Could you check a few things on this model? Use its own coordinates, in mm. Round coordinates to 2 decimals unless told otherwise and drop trailing zeros. Write each loop counter-clockwise with the first axis right and the second up, starting at its lowest first coordinate (ties: lowest second). Pieces come first, ordered by that corner, then holes. Notation, with made-up numbers: (88, -15.75) -> (99, -15.75) arc R16 ccw to (99, 7.25) -> close; hole circle Ø10 at (-14.5, -23.75). An arc over 180 degrees is marked (long way). Answer as CSV lines item,"result". Start each with the question number.
Q1. Imagine slicing it at A-A on z = -445. Please give me the cut outline in (x, y).
Q2. Imagine slicing it at C-C on y = -711.5. Please give me the cut outline in (x, z), and give its area (3 significant figures).
Q3. If I drill on line 1 (Z direction, x = 224.5, y = -403); line 2 (Y direction, x = 148, z = -332); line 3 (Y direction, x = 464.5, z = -278), over which ranges is the centre line in solid material (lowest first)? Write a range as [from, to].
Q4. Imagine slicing it at B-B on x = 1190.5. Please give me the cut outline in (y, z).
Q5. Will these pins go through, and if not, where does the flat tip stop? pin 1 Ø19 at (y, z) = (-130, -216.5) entering from -X; pin 2 Ø19 at (x, z) = (129, -410.5) entering from +Y; pin 3 Ø11.5 at (x, z) = (1260.5, -521.5) entering from -Y.
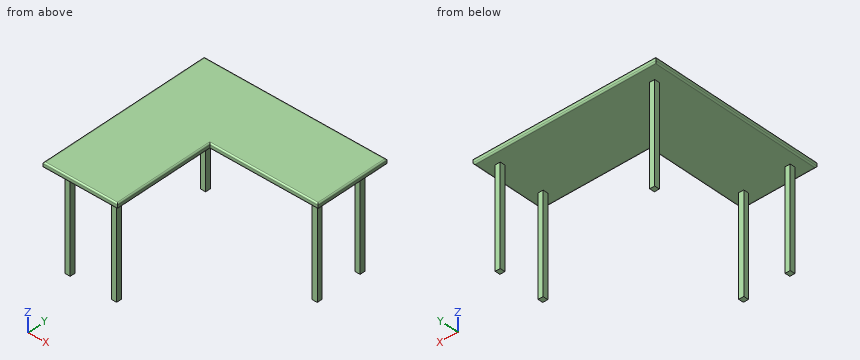
from build123d import *

# Parameters (mm, degrees)
F1_DEPTH = 38.1
F2_R     = 10.16
F3_W     = 38.1
F3_H     = 38.1
F4_DEPTH = 736.6


with BuildPart() as f1:
    # F0 (on Top) → F1 (new body)
    with BuildSketch(Plane.XY):
        Polygon((1371.6, 0), (0, 0), (0, -1308.1), (558.8, -1308.1), (558.8, -558.8), (1371.6, -558.8), align=None)
    extrude(amount=F1_DEPTH)

    # F2
    f2_edges = [f1.edges().sort_by_distance(p)[0] for p in [
        (0, -654.05, 38.1),
        (279.4, -1308.1, 38.1),
        (558.8, -933.45, 38.1),
        (965.2, -558.8, 38.1),
        (1371.6, -279.4, 38.1),
        (685.8, 0, 38.1),
        (279.4, -1308.1, 0),
        (0, -654.05, 0),
        (685.8, 0, 0),
        (1371.6, -279.4, 0),
        (965.2, -558.8, 0),
        (558.8, -933.45, 0),
    ]]
    fillet(f2_edges, radius=F2_R)

    # F3 (on face) → F4 (join)
    with BuildSketch(Plane(origin=(0, 0, 0), x_dir=(1, 0, 0), z_dir=(0, 0, -1))):
        with Locations((130.81, 130.81)):
            Rectangle(F3_W, F3_H)
        with Locations((1266.19, 105.41)):
            Rectangle(F3_W, F3_H)
        with Locations((1266.19, 453.39)):
            Rectangle(F3_W, F3_H)
        with Locations((105.41, 1202.69)):
            Rectangle(F3_W, F3_H)
        with Locations((453.39, 1202.69)):
            Rectangle(F3_W, F3_H)
    extrude(amount=F4_DEPTH)


solid = f1.part
Checks:
1,outline,"(86.36, -1221.74) -> (124.46, -1221.74) -> (124.46, -1183.64) -> (86.36, -1183.64) -> close; (111.76, -149.86) -> (149.86, -149.86) -> (149.86, -111.76) -> (111.76, -111.76) -> close; (434.34, -1221.74) -> (472.44, -1221.74) -> (472.44, -1183.64) -> (434.34, -1183.64) -> close; (1247.14, -472.44) -> (1285.24, -472.44) -> (1285.24, -434.34) -> (1247.14, -434.34) -> close; (1247.14, -124.46) -> (1285.24, -124.46) -> (1285.24, -86.36) -> (1247.14, -86.36) -> close"
2,outline,"(0, 10.16) arc R10.16 ccw to (10.16, 0) -> (548.64, 0) arc R10.16 ccw to (558.8, 10.16) -> (558.8, 27.94) arc R10.16 ccw to (548.64, 38.1) -> (10.16, 38.1) arc R10.16 ccw to (0, 27.94) -> close"
2,area,"21,200 mm^2"
3,line 1,"[0, 38.1]"
3,line 2,"[-149.86, -111.76]"
3,line 3,"[-1221.74, -1183.64]"
4,outline,"(-558.8, 10.16) arc R10.16 ccw to (-548.64, 0) -> (-10.16, 0) arc R10.16 ccw to (0, 10.16) -> (0, 27.94) arc R10.16 ccw to (-10.16, 38.1) -> (-548.64, 38.1) arc R10.16 ccw to (-558.8, 27.94) -> close"
5,pin 1,"x = 111.76"
5,pin 2,"y = -111.76"
5,pin 3,"y = -472.44"
